Verification items for the finished model (mm, model axes). A direction names the side the tool comes from. Give positions to 0.01 mm unless a question says otherwise; leave off trailing zeros. Loops run counter-clockwise (first coordinate to the right, second up) from the corner with the lowest first, then second, coordinate; pieces in that order, holes last. Notation, with made-up numbers: M -4,79.5 L 47,79.5 A24 ccw 47,116.5 Z; hole C 41.5,57 d8. An arc over 180 degrees is marked long. Answer in a Markdown table with one row per item.
Autodesk Inventor part; units mm, degrees
ref_plane "YZ Plane" through (0, 0, 0) normal (1, 0, 0) x (0, 1, 0)
ref_plane "XZ Plane" through (0, 0, 0) normal (0, 1, 0) x (-1, 0, 0)
ref_plane "XY Plane" through (0, 0, 0) normal (0, 0, 1) x (1, 0, 0)
sketch "Sketch1" plane through (0, 0, 0) normal (0, 1, 0) x (-1, 0, 0)
  circle A0 centre (0, 0) radius 100
  circle A1 centre (0, 0) radius 80
  circle A2 centre (0, 0) radius 90
  circle A3 centre (0, 0) radius 88
  circle A4 centre (0, 0) radius 92
  arc A5 (88, 0) -> (92, 0) centre (90, 0) ccw
  arc A6 (0, 92) -> (0, 88) centre (0, 90) ccw
  arc A7 (-88, 0) -> (-92, 0) centre (-90, 0) ccw
  arc A8 (0, -92) -> (0, -88) centre (0, -90) ccw
  dimension "d0" = 200
  dimension "d3" = 20
  dimension "d4" = 10
  dimension "d5" = 2
  dimension "d6" = 2
extrude "Extrusion1" add sketch "Sketch1" along normal blind 10 contours A0 | A1 | A6 A3 A7 A2 | A2 A7 A4 A6 | A5 A4 A8 A2 | A2 A8 A3 A5 | A3
sketch "Sketch2" plane through (0, 10, 0) normal (0, 1, 0) x (1, 0, 0)
  line L0 (0, 0) -> (0, -65)
  line L1 (0, -65) -> (0, 65)
  dimension "d7" = 65
  dimension "d8" = 130
hole "Hole1" at (0, 10, 65) at (0, 10, -65) direction (0, -1, 0) diameter 3.242 end through all
sketch "Sketch3" plane through (0, 10, 0) normal (0, 1, 0) x (1, 0, 0)
  point P0 (0, 0)
  point P1 (0, 0)
hole "Hole2" at (0, 10, 0) direction (0, -1, 0) diameter 4 end through all
properties part number "Aufhängung_Drehscheibe"
Item 1: Sectioned sample at C-C (y = 7.25). Record the cut outline in (x, z), and give its area (3 significant figures).
Reported:
| item | result |
|---|---|
| outline | C 0,0 d200; hole M -92,0 A2 ccw -88,0 A88 cw 0,88 A2 ccw 0,92 A92 ccw Z; hole C 0,0 d4; hole C 0,-65 d3.24; hole C 0,65 d3.24; hole M 0,-92 A92 ccw 92,0 A2 ccw 88,0 A88 cw 0,-88 A2 ccw Z |
| area | 30,200 mm^2 |
Item 2: Tool access check on faces 1 (the flat face through (-21, 0, 1)), 2 (the cylindrical face through (64.3, 4.9, -65.8)). Record the directions out of +Z, -Z, +X, -X, +Y, -Y that give a thin tool (end or side, any length) a straight path to the whole face; none if there is none.
Reported:
| item | result |
|---|---|
| face 1 | +Z, -Z, +X, -X, -Y |
| face 2 | +Y, -Y |
Item 3: Go/stop test with flat-tipped pins: pin 1 (1.5 mm diameter, centred on x = -60.5, y = 8, fed in from +Z); pin 2 (6 mm diameter, centred on y = 4, z = 49.5, fed in from -X); pin 3 (1.5 mm diameter, centred on y = 6.5, z = -28.5, fed in from +X). Record where each tip stops, or that it passes through.
Reported:
| item | result |
|---|---|
| pin 1 | stops at z = 80.19 |
| pin 2 | stops at x = -88.53 |
| pin 3 | stops at x = 96.07 |
Item 4: Scan lines: L1, parallel to Z at x = 0, y = 6.25; L2, parallel to X at y = 3.5, z = 65; L3, parallel to X at y = 2.5, z = -65. Record each from-to range of solid material in increasing order. Write a range as [from, to].
Reported:
| item | result |
|---|---|
| L1 | z = [-100, -92], [-88, -66.62], [-63.38, -2], [2, 63.38], [66.62, 88], [92, 100] |
| L2 | x = [-75.99, -65.11], [-59.32, -1.62], [1.62, 75.99] |
| L3 | x = [-75.99, -1.62], [1.62, 59.32], [65.11, 75.99] |
Item 5: Sectioned sample at B-B (z = -21.5). Record the cut outline in (x, y).
Reported:
| item | result |
|---|---|
| outline | M -97.66,0 L 85.33,0 L 85.33,10 L -97.66,10 Z; M 89.45,0 L 97.66,0 L 97.66,10 L 89.45,10 Z |
Item 6: Sectioned sample at A-A (x = -80). Record the cut outline in (y, z).
Reported:
| item | result |
|---|---|
| outline | M 0,-60 L 10,-60 L 10,36.66 L 0,36.66 Z; M 0,45.43 L 10,45.43 L 10,60 L 0,60 Z |
Item 7: Release check for a two-part mould opening along X. For faces 3 (the cylindrical face through (-61.537, 4.93, 62.906)), 4 (the flat face through (-21, 10, 1)), 5 (the cylindrical face through (-95.38, 4.93, -30.04)) record: released by +X, released by -X, zero draft, split by the parting line, or undercut.
Reported:
| item | result |
|---|---|
| face 3 | undercut |
| face 4 | zero draft |
| face 5 | split by the parting line |
